Source: CAD feature listing. Evaluate the final solid. Frame: model axes, mm. A direction names the side the tool comes from. Round coordinates to 2 decimals unless told otherwise and drop trailing zeros. Write each loop counter-clockwise with the first axis right and the second up, starting at its lowest first coordinate (ties: lowest second). Pieces come first, ordered by that corner, then holes. Notation, with made-up numbers: M 24,83 L 70,83 A16 ccw 70,100 Z; hole C -28,66 d7. An arc over 180 degrees is marked long. Answer in a Markdown table with one row per item. Add a question column.
Item 1: Cut plane C-C on z = 12. Return loops of the section in (x, y).
Item 2: Cut plane A-A on y = 13. Give the number of separate pieces and of enclosed holes in the cut face, and give its area (3 significant figures).
Item 3: Cut plane B-B on z = 5. Return loops of the section in (x, y).
Item 4: Material intervals for probe 1 along X at (y, z) = (18.75, 22.5); probe 2 along Z at (x, y) = (-57.5, 12); probe 3 along X at (y, z) = (12.5, -11), sorted ascending.
Item 5: Mould query, pull axis Z, two halves, no side actions, for faces 1 (the face through (-52.811, 1.521, -11.997)), 2 (the face through (21.379, 13, 30)). Classes: released by +Z, released by -Z, zero draft, split by the parting line, or undercut.
Item 6: Contact query for flat-ended pins moving along their axis: pin 1 (1 mm diameter, centred on x = -97.5, y = 17, fed in from -Z); pin 2 (6 mm diameter, centred on x = -46.5, z = 8.5, fed in from +Y); pin 3 (5 mm diameter, centred on x = 10.88, z = 25.59, fed in from +Y). Output: stop coordinate, or through.
Item 7: Set-up query: faces 3 (the face through (-38.621, 11, -24)), 4 (the face through (-88, 8, -20)), 5 (the face through (11.379, 13, 30)), 6 (the face through (34, 13, 7.591)), 7 (the face through (-37.12, 11.11, 25.55)). Return all of +Z, -Z, +X, -X, +Y, -Y with unobstructed straight access to the full face (end or side cutting, diameter ignored); none if empty.
from build123d import *

# Parameters (mm, degrees)
SKETCH1_W               = 158
SKETCH1_H               = 50
BOSS_EXTRUDE1_DEPTH     = 3
SKETCH2_R               = 1.5
SKETCH2_R_2             = 1.25
CUT_EXTRUDE1_DEPTH      = 4
SKETCH4_W               = 74
SKETCH4_H               = 3.5
BOSS_EXTRUDE2_DEPTH     = 3
SKETCH5_R               = 1.5
CUT_EXTRUDE3_DEPTH      = 4
SKETCH6_W               = 84
SKETCH6_H               = 3
SKETCH6_W_2             = 8
SKETCH6_W_3             = 2
SKETCH6_H_2             = 7
SKETCH6_W_4             = 4
SKETCH6_W_5             = 3
SKETCH6_H_3             = 21
SKETCH6_H_4             = 18
SKETCH6_W_6             = 10
BOSS_EXTRUDE3_DEPTH     = 18
SKETCH8_W               = 10
SKETCH8_H               = 3
SKETCH8_H_2             = 2
SKETCH8_W_2             = 42
SKETCH8_W_3             = 3
SKETCH8_H_3             = 12
BOSS_EXTRUDE4_DEPTH     = 3
CUT_EXTRUDE4_REACH      = 55.5
SKETCH9_W               = 20
SKETCH9_H               = 10
CUT_EXTRUDE5_REACH      = 160
SKETCH10_R              = 1.25
SKETCH11_R              = 1.25
CUT_EXTRUDE6_DEPTH      = 54.5
SKETCH12_R              = 1.25
CUT_EXTRUDE7_DEPTH      = 58
SKETCH13_W              = 10
SKETCH13_H              = 1.5
CUT_EXTRUDE8_DEPTH      = 1.5
SKETCH14_R              = 3
CUT_EXTRUDE9_DEPTH      = 19
CUT_EXTRUDE9_DEPTH_BACK = 0.5
SKETCH15_R              = 3
CUT_EXTRUDE10_DEPTH     = 1
SKETCH17_W              = 1
SKETCH17_H              = 44
BOSS_EXTRUDE5_DEPTH     = 18


with BuildPart() as part:
    # Sketch1 → Boss-Extrude1 (new body)
    with BuildSketch(Plane(origin=(0, 0, 0), x_dir=(1, 0, 0), z_dir=(0, 1, 0))):
        with Locations((-43.62052506, -3.090692124)):
            Rectangle(SKETCH1_W, SKETCH1_H)
    extrude(amount=BOSS_EXTRUDE1_DEPTH)

    # Sketch2 → Cut-Extrude1 (cut, through all)
    with BuildSketch(Plane(origin=(0, 3, 0), x_dir=(1, 0, 0), z_dir=(0, 1, 0))):
        with Locations((-75.12052506, 12.159307876)):
            Circle(SKETCH2_R)
        with Locations((-75.12052506, -18.340692124)):
            Circle(SKETCH2_R)
        with Locations((-44.62052506, -18.340692124)):
            Circle(SKETCH2_R)
        with Locations((-44.62052506, 12.159307876)):
            Circle(SKETCH2_R)
        with Locations((7.87947494, -16.590692124)):
            Circle(SKETCH2_R)
        with Locations((7.87947494, 10.409307876)):
            Circle(SKETCH2_R)
        with Locations((-111.62052506, -19.090692124)):
            Circle(SKETCH2_R)
        with Locations((-111.62052506, 12.909307876)):
            Circle(SKETCH2_R)
        with Locations((-97.62052506, 11.909307876)):
            Circle(SKETCH2_R_2)
        with Locations((-97.62052506, -18.090692124)):
            Circle(SKETCH2_R_2)
        with Locations((-51.62052506, 12.909307876)):
            Circle(SKETCH2_R)
        with Locations((-51.62052506, -19.090692124)):
            Circle(SKETCH2_R)
    extrude(amount=-CUT_EXTRUDE1_DEPTH, mode=Mode.SUBTRACT)

    # Sketch4 → Boss-Extrude2 (add)
    with BuildSketch(Plane(origin=(0, 3, 0), x_dir=(1, 0, 0), z_dir=(0, 1, 0))):
        with Locations((-1.62052506, -29.840692124)):
            Rectangle(SKETCH4_W, SKETCH4_H)
        with Locations((-1.62052506, 23.659307876)):
            Rectangle(SKETCH4_W, SKETCH4_H)
    extrude(amount=-BOSS_EXTRUDE2_DEPTH)

    # Sketch5 → Cut-Extrude3 (cut, through all)
    with BuildSketch(Plane(origin=(0, 3, 0), x_dir=(1, 0, 0), z_dir=(0, 1, 0))):
        with Locations((-34.12052506, 19.409307876)):
            Circle(SKETCH5_R)
        with Locations((-34.12052506, -25.590692124)):
            Circle(SKETCH5_R)
        with Locations((10.87947494, 19.409307876)):
            Circle(SKETCH5_R)
        with Locations((10.87947494, -25.590692124)):
            Circle(SKETCH5_R)
    extrude(amount=-CUT_EXTRUDE3_DEPTH, mode=Mode.SUBTRACT)

    # Sketch6 → Boss-Extrude3 (add)
    with BuildSketch(Plane(origin=(0, 3, 0), x_dir=(1, 0, 0), z_dir=(0, 1, 0))):
        Polygon((35.37947494, 25.409307876), (31.37947494, 25.409307876), (31.37947494, 22.409307876), (32.37947494, 22.409307876), (35.37947494, 22.409307876), align=None)
        with Locations((-80.62052506, -26.590692124)):
            Rectangle(SKETCH6_W, SKETCH6_H)
        with Locations((-80.62052506, 20.409307876)):
            Rectangle(SKETCH6_W, SKETCH6_H)
        with Locations((-34.62052506, 23.909307876)):
            Rectangle(SKETCH6_W_2, SKETCH6_H)
        with Locations((-34.62052506, -30.090692124)):
            Rectangle(SKETCH6_W_2, SKETCH6_H)
        with Locations((-37.62052506, -25.090692124)):
            Rectangle(SKETCH6_W_3, SKETCH6_H_2)
        with Locations((-37.62052506, 18.909307876)):
            Rectangle(SKETCH6_W_3, SKETCH6_H_2)
        with Locations((33.37947494, -30.090692124)):
            Rectangle(SKETCH6_W_4, SKETCH6_H)
        with Locations((33.87947494, -18.090692124)):
            Rectangle(SKETCH6_W_5, SKETCH6_H_3)
        with Locations((33.87947494, 13.409307876)):
            Rectangle(SKETCH6_W_5, SKETCH6_H_4)
        with Locations((16.37947494, -30.090692124)):
            Rectangle(SKETCH6_W_6, SKETCH6_H)
        with Locations((16.37947494, 23.909307876)):
            Rectangle(SKETCH6_W_6, SKETCH6_H)
    extrude(amount=BOSS_EXTRUDE3_DEPTH)

    # Sketch8 → Boss-Extrude4 (add)
    with BuildSketch(Plane(origin=(0, 3, 0), x_dir=(1, 0, 0), z_dir=(0, 1, 0))):
        with Locations((26.37947494, -30.090692124)):
            Rectangle(SKETCH8_W, SKETCH8_H)
        with Locations((26.37947494, 24.409307876)):
            Rectangle(SKETCH8_W, SKETCH8_H_2)
        with Locations((-9.62052506, 23.909307876)):
            Rectangle(SKETCH8_W_2, SKETCH8_H)
        with Locations((-9.62052506, -30.090692124)):
            Rectangle(SKETCH8_W_2, SKETCH8_H)
        with Locations((33.87947494, -1.590692124)):
            Rectangle(SKETCH8_W_3, SKETCH8_H_3)
    extrude(amount=BOSS_EXTRUDE4_DEPTH)

    # Sketch9 → Cut-Extrude4 (cut, up to next)
    with BuildSketch(Plane(origin=(0, 0, -21.909307876), x_dir=(-1, 0, 0), z_dir=(0, 0, -1)), mode=Mode.PRIVATE) as cut_extrude4_sk1:
        with Locations((88.62052506, 13)):
            Rectangle(SKETCH9_W, SKETCH9_H)
    cut_extrude4_tool1 = extrude(cut_extrude4_sk1.sketch, amount=-CUT_EXTRUDE4_REACH, mode=Mode.PRIVATE) & part.part
    add(cut_extrude4_tool1.solids().sort_by_distance((-88.620525, 13, -21.909308))[0], mode=Mode.SUBTRACT)

    # Sketch10 → Cut-Extrude5 (cut, up to next)
    with BuildSketch(Plane(origin=(35.37947494, 0, 0), x_dir=(0, 0, -1), z_dir=(1, 0, 0)), mode=Mode.PRIVATE) as cut_extrude5_sk1:
        with Locations((-21.590692124, 16)):
            Circle(SKETCH10_R)
    cut_extrude5_tool1 = extrude(cut_extrude5_sk1.sketch, amount=-CUT_EXTRUDE5_REACH, mode=Mode.PRIVATE) & part.part
    add(cut_extrude5_tool1.solids().sort_by_distance((35.379475, 16, 21.590692))[0], mode=Mode.SUBTRACT)
    # Sketch10 → Cut-Extrude5 (cut, up to next)
    with BuildSketch(Plane(origin=(35.37947494, 0, 0), x_dir=(0, 0, -1), z_dir=(1, 0, 0)), mode=Mode.PRIVATE) as cut_extrude5_sk2:
        with Locations((15.409307876, 16)):
            Circle(SKETCH10_R)
    cut_extrude5_tool2 = extrude(cut_extrude5_sk2.sketch, amount=-CUT_EXTRUDE5_REACH, mode=Mode.PRIVATE) & part.part
    add(cut_extrude5_tool2.solids().sort_by_distance((35.379475, 16, -15.409308))[0], mode=Mode.SUBTRACT)

    # Sketch11 → Cut-Extrude6 (cut, through all)
    with BuildSketch(Plane(origin=(0, 0, -21.909307876), x_dir=(-1, 0, 0), z_dir=(0, 0, -1))):
        with Locations((43.62052506, 16)):
            Circle(SKETCH11_R)
        with Locations((110.12052506, 16)):
            Circle(SKETCH11_R)
        with Locations((52.62052506, 16)):
            Circle(SKETCH11_R)
        with Locations((101.12052506, 16)):
            Circle(SKETCH11_R)
    extrude(amount=-CUT_EXTRUDE6_DEPTH, mode=Mode.SUBTRACT)

    # Sketch12 → Cut-Extrude7 (cut, through all)
    with BuildSketch(Plane(origin=(0, 0, -25.409307876), x_dir=(-1, 0, 0), z_dir=(0, 0, -1))):
        with Locations((34.62052506, 16)):
            Circle(SKETCH12_R)
    extrude(amount=-CUT_EXTRUDE7_DEPTH, mode=Mode.SUBTRACT)

    # Sketch13 → Cut-Extrude8 (cut)
    with BuildSketch(Plane(origin=(0, 0, 0), x_dir=(-1, 0, 0), z_dir=(0, -1, 0))):
        with Locations((33.62052506, -30.840692124)):
            Rectangle(SKETCH13_W, SKETCH13_H)
        with Locations((33.62052506, 24.659307876)):
            Rectangle(SKETCH13_W, SKETCH13_H)
    extrude(amount=-CUT_EXTRUDE8_DEPTH, mode=Mode.SUBTRACT)

    # Sketch14 → Cut-Extrude9 (cut, two sides)
    with BuildSketch(Plane(origin=(0, 3, 0), x_dir=(1, 0, 0), z_dir=(0, 1, 0))) as cut_extrude9_sk:
        with Locations((10.87947494, -25.590692124)):
            Circle(SKETCH14_R)
        with Locations((-34.12052506, -25.590692124)):
            Circle(SKETCH14_R)
        with Locations((-34.12052506, 19.409307876)):
            Circle(SKETCH14_R)
        with Locations((10.87947494, 19.409307876)):
            Circle(SKETCH14_R)
    extrude(amount=CUT_EXTRUDE9_DEPTH, mode=Mode.SUBTRACT)
    extrude(cut_extrude9_sk.sketch, amount=-CUT_EXTRUDE9_DEPTH_BACK, mode=Mode.SUBTRACT)

    # Sketch15 → Cut-Extrude10 (cut)
    with BuildSketch(Plane(origin=(0, 3, 0), x_dir=(1, 0, 0), z_dir=(0, 1, 0))):
        with Locations((-75.12052506, 12.159307876)):
            Circle(SKETCH15_R)
        with Locations((-75.12052506, -18.340692124)):
            Circle(SKETCH15_R)
        with Locations((-44.62052506, 12.159307876)):
            Circle(SKETCH15_R)
        with Locations((-44.62052506, -18.340692124)):
            Circle(SKETCH15_R)
    extrude(amount=-CUT_EXTRUDE10_DEPTH, mode=Mode.SUBTRACT)

    # Sketch17 → Boss-Extrude5 (add)
    with BuildSketch(Plane(origin=(0, 3, 0), x_dir=(1, 0, 0), z_dir=(0, 1, 0))):
        with Locations((-122.12052506, -3.090692124)):
            Rectangle(SKETCH17_W, SKETCH17_H)
    extrude(amount=BOSS_EXTRUDE5_DEPTH)


solid = part.part
Results below:
| question | item | result |
|---|---|---|
| 1 | outline | M -122.62,0 L 35.38,0 L 35.38,21 L 32.38,21 L 32.38,3 L -121.62,3 L -121.62,21 L -122.62,21 Z |
| 2 | separate pieces | 6 |
| 2 | enclosed holes | 0 |
| 2 | area | 763 mm2 |
| 3 | outline | M -122.62,0 L 35.38,0 L 35.38,6 L 32.38,6 L 32.38,3 L -121.62,3 L -121.62,21 L -122.62,21 Z |
| 4 | probe 1 | -122.62 to -121.62, -38.62 to -36.62, 32.38 to 35.38 |
| 4 | probe 2 | -21.91 to -18.91, 25.09 to 28.09 |
| 4 | probe 3 | -122.62 to -121.62, 32.38 to 35.38 |
| 5 | face 1 | undercut |
| 5 | face 2 | zero draft |
| 6 | pin 1 | z = 25.09 |
| 6 | pin 2 | y = 3 |
| 6 | pin 3 | y = 2.5 |
| 7 | face 3 | -Z, -X, +Y, -Y |
| 7 | face 4 | -Z |
| 7 | face 5 | +Z, -Z, +Y |
| 7 | face 6 | +X, +Y |
| 7 | face 7 | +Y |
